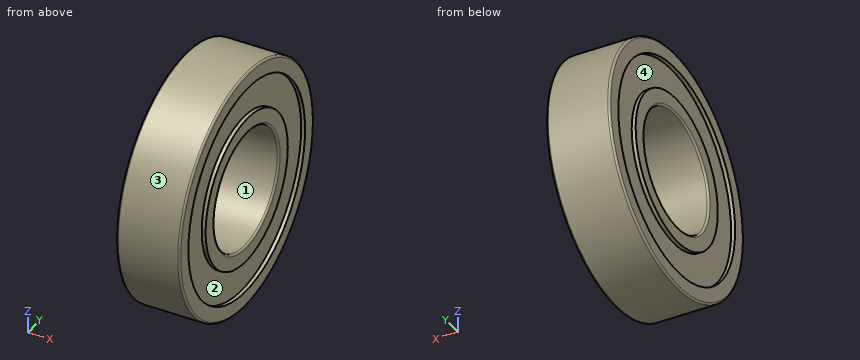
```python
from build123d import *

# Parameters (mm, degrees)
FILLET_R = 0.5


with BuildPart() as part:
    # Sketch → Revolution (revolve)
    with BuildSketch(Plane.XY):
        Polygon((-2.138438, 31), (-18.138438, 31), (-18.138438, 27), (-17.138438, 27), (-17.138438, 19), (-18.138438, 19), (-18.138438, 15), (-2.138438, 15), (-2.138438, 19), (-3.138438, 19), (-3.138438, 27), (-2.138438, 27), align=None)
    revolve(axis=Axis((0, 0, 0), (1, 0, 0)))

    # Fillet
    fillet_edges = [part.edges().sort_by_distance(p)[0] for p in [
        (-2.138438, -31, 0),
        (-2.138438, -15, 0),
        (-18.138438, -31, 0),
        (-18.138438, -15, 0),
    ]]
    fillet(fillet_edges, radius=FILLET_R)


solid = part.part
```
Model file for the job. Use its own axes, mm. Face numbers are marked on the shaded views. A direction names the side the tool comes from. Coordinates: 2 decimals unless noted, no trailing zeros. Loops run counter-clockwise (first coordinate to the right, second up) from the corner with the lowest first, then second, coordinate; pieces in that order, holes last. Notation, with made-up numbers: (6.25, -36.5) -> (61.25, -36.5) arc R21 cw to (61.25, -26.5) -> close; hole circle Ø4 at (80, 48.5). An arc over 180 degrees is marked (long way). Answer as a JSON object with one key per item and string values.
Q1. Probe probe 1 along Z at (x, y) = (-2.6, 0); probe 2 along Z at (x, y) = (-13, 0); probe 3 along Y at (x, z) = (-8.75, 24.5). List the from-to ranges inside material, lowest first.
Report:
{"probe 1": "z = -31 to -27, -19 to -15, 15 to 19, 27 to 31", "probe 2": "z = -31 to -15, 15 to 31", "probe 3": "y = -18.99 to 18.99"}
Q2. 3-axis set-ups, long thin cutter, end or side, ignore diameter. For the marked faces 1 and 2: which of +Z, -Z, +X, -X, +Y, -Y reach the whole face in a straight line?
Report:
{"face 1": "+X, -X", "face 2": "+X"}
Q3. Cut at B-B (x = -15). List the corners of the cut face in (y, z), and give its area (3 significant figures).
Report:
{"outline": "circle Ø62 at (0, 0); hole circle Ø30 at (0, 0)", "area": "2,310 mm2"}
Q4. Flat gauge pins, fed straight in: P1, Ø4, axis at x = -8.5, z = -21, coming from the -Y side; P2, Ø4, axis at x = -8.5, y = -12.5, coming from the +Z side; P3, Ø1.5, axis at x = -5, z = 16.5, coming from the +Y side. Where does each tip first touch, or does it go through?
Report:
{"P1": "stops at y = -24.49", "P2": "stops at z = 29.17", "P3": "stops at y = 26.7"}
Q5. Pull direction Z, two halves, no side cores. Call the marked faces 3 and 4: released by +Z, released by -Z, zero draft, split by the parting line, or undercut.
Report:
{"face 3": "split by the parting line", "face 4": "undercut"}
